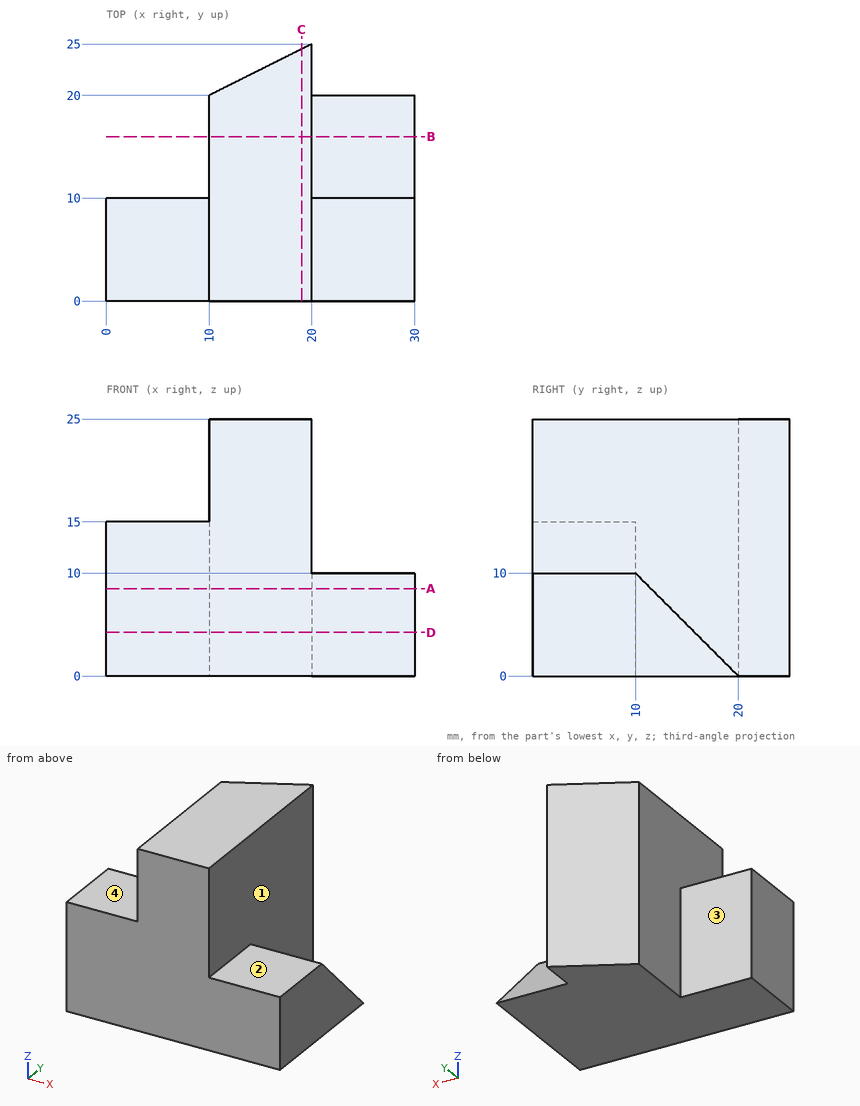
Geometry check sheet. Reference: drawing and pictorial views, mm from the part's lowest x, y, z. A direction names the side the tool comes from. Coordinates: 2 decimals unless noted, no trailing zeros. Order: outer loops, then holes, each group sorted by start corner. A loop starts at its lowest first (then second) coordinate and runs counter-clockwise, first axis right, second up. Notation, with made-up numbers: (36, 56.5) -> (60, 56.5) arc R29 cw to (60, 91.5) -> close; hole circle Ø4 at (-39.75, 16.25). An arc over 180 degrees is marked (long way). Put each result on its own line as item: value. Start each with the question number.
1) Go/stop test with flat-tipped pins: pin 1 (6 mm diameter, centred on y = 20, z = 7.5, fed in from -X); pin 2 (6 mm diameter, centred on x = 25, y = 6.5, fed in from +Z); pin 3 (5 mm diameter, centred on x = 4.5, y = 3.5, fed in from +Z). Record where each tip stops, or that it passes through.
2) Cross-section at A-A (z = 8.5). Enter the section's corners in (x, y), plus the area to 3 significant figures.
3) Cross-section at D-D (z = 4.25). Enter the section's corners in (x, y), plus the area to 4 significant figures.
4) Cross-section at C-C (x = 19). Enter the section's corners in (y, z), plus the area to 4 significant figures.
5) Tool access check on the marked faces 1, 2, 3 and 4. Record the directions out of +Z, -Z, +X, -X, +Y, -Y that give a thin tool (end or side, any length) a straight path to the whole face; none if there is none.
6) Material ranges on L1, parallel to X at y = 19.25, z = 2; L2, parallel to X at y = 12, z = 2.5; L3, parallel to Z at x = 28.75, y = 1, recorded low to high.
7) Cross-section at B-B (y = 16). Enter the section's corners in (x, z).
Geometry check:
1. pin 1: stops at x = 10
1. pin 2: stops at z = 10
1. pin 3: stops at z = 15
2. outline: (0, 0) -> (30, 0) -> (30, 11.5) -> (20, 11.5) -> (20, 25) -> (10, 20) -> (10, 10) -> (0, 10) -> close
2. area: 440 mm^2
3. outline: (0, 0) -> (30, 0) -> (30, 15.75) -> (20, 15.75) -> (20, 25) -> (10, 20) -> (10, 10) -> (0, 10) -> close
3. area: 482.5 mm^2
4. outline: (0, 0) -> (24.5, 0) -> (24.5, 25) -> (0, 25) -> close
4. area: 612.5 mm^2
5. face 1: +Z, +X, +Y
5. face 2: +Z, +X, +Y, -Y
5. face 3: +Z, -Z, -X, +Y
5. face 4: +Z, -X, +Y, -Y
6. L1: x = 10 to 20
6. L2: x = 10 to 30
6. L3: z = 0 to 10
7. outline: (10, 0) -> (30, 0) -> (30, 4) -> (20, 4) -> (20, 25) -> (10, 25) -> close
